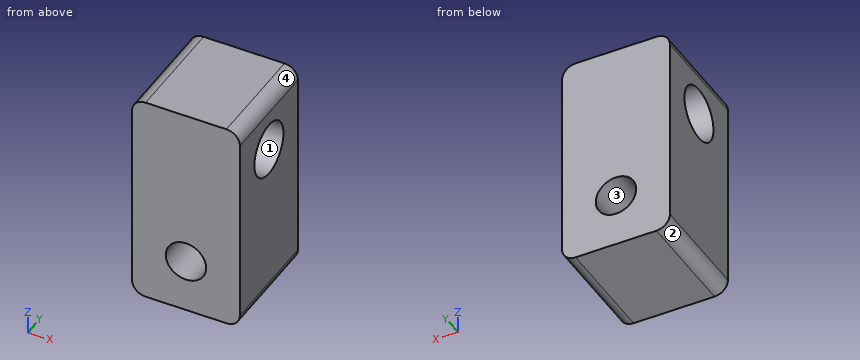
from build123d import *

# Parameters (mm, degrees)
F1_DEPTH = 25.4
F2_R     = 6.35
F3_DEPTH = 25.4
F4_R     = 4.7625
F5_DEPTH = 25.4


with BuildPart() as f1:
    # F0 (on Front) → F1 (new body)
    with BuildSketch(Plane.XZ):
        with BuildLine():
            ThreePointArc((-20.750085, -26.389282), (-19.820149, -28.634346), (-17.575085, -29.564282))
            Line((-17.575085, -29.564282), (1.474915, -29.564282))
            ThreePointArc((1.474915, -29.564282), (3.719979, -28.634346), (4.649915, -26.389282))
            Line((4.649915, -26.389282), (4.649915, 18.060718))
            ThreePointArc((4.649915, 18.060718), (3.719979, 20.305782), (1.474915, 21.235718))
            Line((1.474915, 21.235718), (-17.575085, 21.235718))
            ThreePointArc((-17.575085, 21.235718), (-19.820149, 20.305782), (-20.750085, 18.060718))
            Line((-20.750085, 18.060718), (-20.750085, -26.389282))
        make_face()
    extrude(amount=F1_DEPTH)

    # F2 (on face) → F3 (cut)
    with BuildSketch(Plane.YZ.offset(4.649915)):
        with Locations((-12.7, 8.535718)):
            Circle(F2_R)
    extrude(amount=-F3_DEPTH, mode=Mode.SUBTRACT)

    # F4 (on face) → F5 (cut)
    with BuildSketch(Plane(origin=(0, 0, 0), x_dir=(-1, 0, 0), z_dir=(0, 1, 0))):
        with Locations((8.050085, -16.864282)):
            Circle(F4_R)
    extrude(amount=-F5_DEPTH, mode=Mode.SUBTRACT)


solid = f1.part
Source: CAD feature listing. Evaluate the final solid. Frame: model axes, mm. Face numbers are marked on the shaded views. Give positions to 0.01 mm unless a question says otherwise; leave off trailing zeros. Write each loop counter-clockwise with the first axis right and the second up, starting at its lowest first coordinate (ties: lowest second). Pieces come first, ordered by that corner, then holes. Notation, with made-up numbers: M -2,9.25 L 9,9.25 A23 ccw 9,41.25 Z; hole C 56,54 d6. An arc over 180 degrees is marked long. Return JSON: item names as keys, results as strings. Group by question number.
1) Cut plane B-B, the plane z = -19. Output: boundary loops of the cut face in (x, y), plus the area to 3 significant figures.
2) Cut plane A-A, the plane y = -7.75. Give the number of separate pieces and of enclosed holes in the cut face, plus the area to 3 significant figures.
3) Material intervals for line 1 along Z through (x, y) = (-2.25, -12.7); line 2 along Z through (x, y) = (-6.75, -12.7); line 3 along Y through (x, z) = (-12.5, 10), sorted ascending. Write a range as [from, to].
4) Pin query (flat end, axial travel): P1, Ø1.5, axis at x = -3, z = -23.5, coming from the +Y side. Return the tip coordinate at first contact, or that it passes through.
5) Pull-direction query (X, two-part tool) for the marked faces 1, 2, 3 and 4; classes: pulls with the +X half, pulls with the -X half, needs draft (parallel to the pull), parting line crosses it, or undercut.
6) Cut plane C-C, the plane x = -8. Output: boundary loops of the cut face in (y, z), plus the area to 3 significant figures.
Recorded:
{
 "1": {"outline": "M -20.75,-25.4 L -12.31,-25.4 L -12.31,0 L -20.75,0 Z; M -3.79,-25.4 L 4.65,-25.4 L 4.65,0 L -3.79,0 Z", "area": "429 mm²"},
 "2": {"separate pieces": "2", "enclosed holes": "1", "area": "1,010 mm²"},
 "3": {"line 1": "z = [-29.56, 2.19], [14.89, 21.24]", "line 2": "z = [-29.56, -21.45], [-12.28, 2.19], [14.89, 21.24]", "line 3": "y = [-25.4, -18.88], [-6.52, 0]"},
 "4": {"P1": "stops at y = 0"},
 "5": {"face 1": "needs draft", "face 2": "pulls with the -X half", "face 3": "undercut", "face 4": "pulls with the +X half"},
 "6": {"outline": "M -25.4,-29.56 L 0,-29.56 L 0,-21.63 L -25.4,-21.63 Z; M -25.4,-12.1 L 0,-12.1 L 0,21.24 L -25.4,21.24 Z; hole C -12.7,8.54 d12.7", "area": "922 mm²"}
}
